The listing builds one solid part. Answer for the finished solid, in the listing's coordinates (mm). Give positions to 0.01 mm unless a question says otherwise; leave off trailing zeros. Loops run counter-clockwise (first coordinate to the right, second up) from the corner with the lowest first, then second, coordinate; pieces in that order, holes last. Notation, with made-up numbers: M 13,-12 L 34,-12 A27 ccw 34,10 Z; hole C 68,-33.75 d9. An arc over 180 degrees is marked long. One line per item, written item: value. Start each with the question number.
Q1. The mould has two halves that part along X. Classify faces 1 (the flat face through (0, -24, 0)), 2 (the flat face through (0, -22.225, 155)), 3 (the flat face through (19.05, -13, 150)), 4 (the flat face through (-15.457, -3.494, 150.266)): +X half, -X half, draft (parallel to the pull), parting line (faces both ways), or undercut.
Q2. Consider L1, parallel to Y at x = 15.5, z = 223.5; L2, parallel to X at y = -7.5, z = 146; L3, parallel to X at y = -7, z = 104. Determine where each line is inside the solid, lowest interval first.
Q3. A cutting plane is placed at A-A, the plane x = 4.5. Determine the outline of the cut face in (y, z) (3 decimals).
Q4. A cutting plane is placed at B-B, the plane z = 235.5. State how many separate pieces and enclosed holes the cut face has, and give its area (3 significant figures).
Q5. Flat-ended cylindrical pins translate along their axes: pin 1 (1 mm diameter, centred on x = 14, z = 156, fed in from -Y); pin 2 (2.5 mm diameter, centred on x = -12.7, y = -19.05, fed in from +Z). Find the tip coordinate at first contact, or state that the pin passes through.
from build123d import *

# Parameters (mm, degrees)
F0_R     = 1.35255
F1_DEPTH = 304.8
F2_T     = 3.175
F3_DEPTH = 3.175
F5_DEPTH = 304.8


# Not quite as in the source:
# - a pattern or mirror of a feature is missing from the dataset's text; its kind, count and spacing are read off the source's solid
# - a shell that OpenCascade refuses in one call is made with other operations: the cavity is built on its own and cut out


with BuildPart() as f1:
    # F0 (on Top) → F1 (new body)
    with BuildSketch(Plane.XY):
        Polygon((11.9626600757, 0), (-11.9626600757, 0), (-19.05, -7.0873399243), (-19.05, -18.3126600757), (-11.9626600757, -25.4), (11.9626600757, -25.4), (19.05, -18.3126600757), (19.05, -7.0873399243), align=None)
        with Locations((-12.7, -19.05)):
            Circle(F0_R, mode=Mode.SUBTRACT)
        with Locations((12.7, -19.05)):
            Circle(F0_R, mode=Mode.SUBTRACT)
        with Locations((-12.7, -6.35)):
            Circle(F0_R, mode=Mode.SUBTRACT)
        with Locations((12.7, -6.35)):
            Circle(F0_R, mode=Mode.SUBTRACT)
    extrude(amount=F1_DEPTH)

    # F2: shell of thickness 3.175, made by hand


with BuildPart() as f2_core1:
    # F2_t2: copy of F1
    add(f1.part)

    # the walls: a layer under each face that stays
    f2_faces = [f2_core1.faces().sort_by_distance(p)[0] for p in [
        (0, 0, 152.4),
        (-15.5063300378, -3.5436699622, 152.4),
        (-19.05, -12.7, 152.4),
        (-15.5063300378, -21.8563300378, 152.4),
        (0, -25.4, 152.4),
        (15.5063300378, -21.8563300378, 152.4),
        (19.05, -12.7, 152.4),
        (15.5063300378, -3.5436699622, 152.4),
        (-14.05255, -19.05, 152.4),
        (11.34745, -19.05, 152.4),
        (-14.05255, -6.35, 152.4),
        (11.34745, -6.35, 152.4),
        (0, -12.7, 0),
    ]]
    thicken(f2_faces, amount=-F2_T, mode=Mode.SUBTRACT)


with BuildPart() as f1_1:
    add(f1.part)

    # what is left inside the walls is the cavity
    f2_cavity = [f2_core1.part.solids().sort_by_distance(p)[0] for p in [
        (0, -3.20675, 204.258333),
    ]]
    add(f2_cavity, mode=Mode.SUBTRACT)

    # F3 (cut, through all): a face of the model
    f3_faces = [f1_1.faces().sort_by_distance(p)[0] for p in [
        (0, -12.7, 3.175),
    ]]
    extrude(f3_faces, amount=-F3_DEPTH, mode=Mode.SUBTRACT)

    # F4 (on face) → F5 (cut, through all)
    with BuildSketch(Plane.XY.offset(304.8)):
        with BuildLine():
            ThreePointArc((15.5063300378, -9.1563300378), (9.8936699622, -9.1563300378), (9.8936699622, -3.5436699622))
            Line((9.8936699622, -3.5436699622), (10.2623399243, -3.175))
            Line((10.2623399243, -3.175), (9.4722943129, -3.175))
            ThreePointArc((9.4722943129, -3.175), (9.4985386928, -9.5514613072), (15.875, -9.5777056871))
            Line((15.875, -9.5777056871), (15.875, -8.7876600757))
            Line((15.875, -8.7876600757), (15.5063300378, -9.1563300378))
        make_face()
        with BuildLine():
            Line((15.875, -16.6123399243), (15.875, -15.8222943129))
            ThreePointArc((15.875, -15.8222943129), (9.4985386928, -15.8485386928), (9.4722943129, -22.225))
            Line((9.4722943129, -22.225), (10.2623399243, -22.225))
            Line((10.2623399243, -22.225), (9.8936699622, -21.8563300378))
            ThreePointArc((9.8936699622, -21.8563300378), (9.8936699622, -16.2436699622), (15.5063300378, -16.2436699622))
            Line((15.5063300378, -16.2436699622), (15.875, -16.6123399243))
        make_face()
    f5 = extrude(amount=-F5_DEPTH, mode=Mode.SUBTRACT)

    # F5_copies: F5 across plane
    add(f5.mirror(Plane(origin=(0, 0, 0), x_dir=(0, 0, -1), z_dir=(-1, 0, 0))), mode=Mode.SUBTRACT)


solid = f1_1.part
Answer block:
1. face 1: draft
1. face 2: undercut
1. face 3: +X half
1. face 4: -X half
2. L1: -21.86 to -16.24, -9.16 to -3.54
2. L2: -19.05 to -13.41, -11.99 to -8.9, 8.9 to 11.99, 13.41 to 19.05
2. L3: -18.96 to -13.89, -11.51 to -8.78, 8.78 to 11.51, 13.89 to 18.96
3. outline: M -25.4,0 L -22.225,0 L -22.225,304.8 L -25.4,304.8 Z; M -3.175,0 L 0,0 L 0,304.8 L -3.175,304.8 Z
4. separate pieces: 1
4. enclosed holes: 5
4. area: 418 mm^2
5. pin 1: y = -23.86
5. pin 2: through
